```python
from build123d import *

# Parameters (mm, degrees)
F1_DEPTH = 6.35


with BuildPart() as f1:
    # F0 (on Top) → F1 (new body)
    with BuildSketch(Plane.XY):
        with BuildLine():
            Line((35.9444015112, 0.8), (39.9499687109, 0.8))
            ThreePointArc((39.9499687109, 0.8), (0, 38.8), (-39.9499687109, 0.8))
            Line((-39.9499687109, 0.8), (-35.9444015112, 0.8))
            ThreePointArc((-35.9444015112, 0.8), (0, 34.8), (35.9444015112, 0.8))
        make_face()
        with BuildLine():
            Line((-35.9444015112, 0.8), (-39.9499687109, 0.8))
            ThreePointArc((-39.9499687109, 0.8), (-39.9874902215, -0.1996871577), (-40, -1.2))
            ThreePointArc((-40, -1.2), (-39.9874902215, -2.2003128423), (-39.9499687109, -3.2))
            Line((-39.9499687109, -3.2), (-35.9444015112, -3.2))
            ThreePointArc((-35.9444015112, -3.2), (-36, -1.2), (-35.9444015112, 0.8))
        make_face()
        with BuildLine():
            ThreePointArc((-39.9499687109, -3.2), (0, -41.2), (39.9499687109, -3.2))
            Line((39.9499687109, -3.2), (35.9444015112, -3.2))
            ThreePointArc((35.9444015112, -3.2), (0, -37.2), (-35.9444015112, -3.2))
            Line((-35.9444015112, -3.2), (-39.9499687109, -3.2))
        make_face()
        with BuildLine():
            ThreePointArc((39.9499687109, -3.2), (39.9874902215, -2.2003128423), (40, -1.2))
            ThreePointArc((40, -1.2), (39.9874902215, -0.1996871577), (39.9499687109, 0.8))
            Line((39.9499687109, 0.8), (35.9444015112, 0.8))
            ThreePointArc((35.9444015112, 0.8), (35.9860976934, -0.1996136756), (36, -1.2))
            ThreePointArc((36, -1.2), (35.9860976934, -2.2003863244), (35.9444015112, -3.2))
            Line((35.9444015112, -3.2), (39.9499687109, -3.2))
        make_face()
        with BuildLine():
            ThreePointArc((36, -1.2), (35.9860976934, -0.1996136756), (35.9444015112, 0.8))
            Line((35.9444015112, 0.8), (23.9165214862, 0.8))
            ThreePointArc((23.9165214862, 0.8), (23.9791212899, -0.1991292963), (24, -1.2))
            ThreePointArc((24, -1.2), (23.9791212899, -2.2008707037), (23.9165214862, -3.2))
            Line((23.9165214862, -3.2), (35.9444015112, -3.2))
            ThreePointArc((35.9444015112, -3.2), (35.9860976934, -2.2003863244), (36, -1.2))
        make_face()
        with BuildLine():
            ThreePointArc((24, -1.2), (23.9791212899, -0.1991292963), (23.9165214862, 0.8))
            Line((23.9165214862, 0.8), (19.8997487421, 0.8))
            ThreePointArc((19.8997487421, 0.8), (19.9749214622, -0.1987444988), (20, -1.2))
            ThreePointArc((20, -1.2), (19.9749214622, -2.2012555012), (19.8997487421, -3.2))
            Line((19.8997487421, -3.2), (23.9165214862, -3.2))
            ThreePointArc((23.9165214862, -3.2), (23.9791212899, -2.2008707037), (24, -1.2))
        make_face()
        with BuildLine():
            Line((19.8997487421, 0.8), (23.9165214862, 0.8))
            ThreePointArc((23.9165214862, 0.8), (0, 22.8), (-23.9165214862, 0.8))
            Line((-23.9165214862, 0.8), (-19.8997487421, 0.8))
            ThreePointArc((-19.8997487421, 0.8), (0, 18.8), (19.8997487421, 0.8))
        make_face()
        with BuildLine():
            Line((-19.8997487421, 0.8), (-23.9165214862, 0.8))
            ThreePointArc((-23.9165214862, 0.8), (-24, -1.2), (-23.9165214862, -3.2))
            Line((-23.9165214862, -3.2), (-19.8997487421, -3.2))
            ThreePointArc((-19.8997487421, -3.2), (-20, -1.2), (-19.8997487421, 0.8))
        make_face()
        with BuildLine():
            Line((-23.9165214862, 0.8), (-35.9444015112, 0.8))
            ThreePointArc((-35.9444015112, 0.8), (-36, -1.2), (-35.9444015112, -3.2))
            Line((-35.9444015112, -3.2), (-23.9165214862, -3.2))
            ThreePointArc((-23.9165214862, -3.2), (-24, -1.2), (-23.9165214862, 0.8))
        make_face()
    extrude(amount=F1_DEPTH)


solid = f1.part
```
CAD build for the part. Positions are in the model's coordinates, mm. A direction names the side the tool comes from. Round coordinates to 2 decimals unless told otherwise and drop trailing zeros. Write each loop counter-clockwise with the first axis right and the second up, starting at its lowest first coordinate (ties: lowest second). Pieces come first, ordered by that corner, then holes.
Item 1: Mould opens along X. For faces 3 (the cylindrical face through (0.76, -37.19, 3.13)), 4 (the flat face through (0, 20, 6.35)), 5 (the flat face through (-28, -3.2, 3)) say: released by +X, released by -X, zero draft, split by the parting line, or undercut.
Filled in:
face 3: undercut
face 4: zero draft
face 5: undercut
Item 2: Band-saw the part on D-D on y = 27.5. Write the cut outline in (x, z), then the cut area to 3 significant figures.
Filled in:
outline: (-27.86, 0) - (-21.73, 0) - (-21.73, 6.35) - (-27.86, 6.35) - close; (21.73, 0) - (27.86, 0) - (27.86, 6.35) - (21.73, 6.35) - close
area: 77.8 mm2
Item 3: Tool access for faces 1 (the cylindrical face through (0.5, 22.795, 3.131)), 2 (the flat face through (0, 20, 0)): list every direction of +Z, -Z, +X, -X, +Y, -Y with a clear straight run to the whole face (end or side of a thin tool).
Filled in:
face 1: +Z, -Z
face 2: -Z, +X, -X, +Y, -Y
Item 4: Drill centre lines: L1, parallel to X at y = 6, z = 3.75; L2, parallel to Y at x = -28.5, z = 1.75; L3, parallel to X at y = 17, z = 5.25. Where is each one in solid material? Low to high.
Filled in:
L1: x = -39.35 to -35.27, -22.89 to -18.66, 18.66 to 22.89, 35.27 to 39.35
L2: y = -29.27 to -23.19, -3.2 to 0.8, 20.79 to 26.87
L3: x = -35.62 to -31.06, -15.64 to -8.29, 8.29 to 15.64, 31.06 to 35.62
Item 5: Band-saw the part on A-A on x = 0. Write the cut outline in (y, z), then the cut area to 3 significant figures.
Filled in:
outline: (-41.2, 0) - (-37.2, 0) - (-37.2, 6.35) - (-41.2, 6.35) - close; (18.8, 0) - (22.8, 0) - (22.8, 6.35) - (18.8, 6.35) - close; (34.8, 0) - (38.8, 0) - (38.8, 6.35) - (34.8, 6.35) - close
area: 76.2 mm2
Item 6: Drop flat-ended pins along their axis: pin 1 Ø6 at (x, y) = (30.5, -22.5) entering from -Z; pin 2 Ø6 at (x, y) = (-7, 27) entering from +Z; pin 3 Ø2 at (x, z) = (-7, 5.5) entering from -Y; pin 4 Ø3 at (x, z) = (-27, 4.5) entering from +Y. Give the stop position or say it passes through.
Filled in:
pin 1: stops at z = 0
pin 2: passes through
pin 3: stops at y = -40.75
pin 4: stops at y = 29.62
Item 7: Band-saw the part on C-C on y = 5. Write the cut outline in (x, z), then the cut area to 3 significant figures.
Filled in:
outline: (-39.52, 0) - (-35.46, 0) - (-35.46, 6.35) - (-39.52, 6.35) - close; (-23.19, 0) - (-19.01, 0) - (-19.01, 6.35) - (-23.19, 6.35) - close; (19.01, 0) - (23.19, 0) - (23.19, 6.35) - (19.01, 6.35) - close; (35.46, 0) - (39.52, 0) - (39.52, 6.35) - (35.46, 6.35) - close
area: 104 mm2
